```python
from build123d import *

# Parameters (mm, degrees)
SKETCH1_W                  = 50.8
SKETCH1_H                  = 76.2
BOSS_EXTRUDE1_DEPTH        = 1.5875
SKETCH2_W                  = 43.942
SKETCH2_H                  = 69.342
BOSS_EXTRUDE2_DEPTH        = 9.525
FILLET1_R                  = 6.35
CUT_EXTRUDE1_DEPTH         = 9.525
F_4_40_TAPPED_HOLE1_REACH  = 79.663
F_4_40_TAPPED_HOLE1_BORE_R = 1.1303
FILLET2_R                  = 1.5875


with BuildPart() as part:
    # Sketch1 → Boss-Extrude1 (new body)
    with BuildSketch(Plane.XY):
        Rectangle(SKETCH1_W, SKETCH1_H)
    extrude(amount=BOSS_EXTRUDE1_DEPTH)

    # Sketch2 → Boss-Extrude2 (add)
    with BuildSketch(Plane(origin=(0, 0, 0), x_dir=(-1, 0, 0), z_dir=(0, 0, -1))):
        Rectangle(SKETCH2_W, SKETCH2_H)
    extrude(amount=BOSS_EXTRUDE2_DEPTH)

    # Fillet1
    fillet1_edges = [part.edges().sort_by_distance(p)[0] for p in [
        (-21.971, -34.671, -4.7625),
        (-21.971, 34.671, -4.7625),
        (21.971, 34.671, -4.7625),
        (21.971, -34.671, -4.7625),
    ]]
    fillet(fillet1_edges, radius=FILLET1_R)

    # Sketch3 → Cut-Extrude1 (cut)
    with BuildSketch(Plane(origin=(0, 0, -9.525), x_dir=(-1, 0, 0), z_dir=(0, 0, -1))):
        with BuildLine():
            Line((-18.796, 28.321), (-18.796, -28.321))
            ThreePointArc((-18.796, -28.321), (-17.86606403, -30.56606403), (-15.621, -31.496))
            Line((-15.621, -31.496), (15.621, -31.496))
            ThreePointArc((15.621, -31.496), (17.86606403, -30.56606403), (18.796, -28.321))
            Line((18.796, -28.321), (18.796, 28.321))
            ThreePointArc((18.796, 28.321), (17.86606403, 30.56606403), (15.621, 31.496))
            Line((15.621, 31.496), (-15.621, 31.496))
            ThreePointArc((-15.621, 31.496), (-17.86606403, 30.56606403), (-18.796, 28.321))
        make_face()
    extrude(amount=-CUT_EXTRUDE1_DEPTH, mode=Mode.SUBTRACT)

    # 4-40 Tapped Hole1 bore → 4-40 Tapped Hole1 (cut, up to next)
    with BuildSketch(Plane(origin=(0, 34.671, 0), x_dir=(-1, 0, 0), z_dir=(0, 1, 0)), mode=Mode.PRIVATE) as f_4_40_tapped_hole1_sk1:
        with Locations((-9.525, -4.7625)):
            Circle(F_4_40_TAPPED_HOLE1_BORE_R)
    f_4_40_tapped_hole1_tool1 = extrude(f_4_40_tapped_hole1_sk1.sketch, amount=-F_4_40_TAPPED_HOLE1_REACH, mode=Mode.PRIVATE) & part.part
    # 4-40 Tapped Hole1 bore → 4-40 Tapped Hole1 (cut, up to next)
    with BuildSketch(Plane(origin=(0, 34.671, 0), x_dir=(-1, 0, 0), z_dir=(0, 1, 0)), mode=Mode.PRIVATE) as f_4_40_tapped_hole1_sk2:
        with Locations((9.525, -4.7625)):
            Circle(F_4_40_TAPPED_HOLE1_BORE_R)
    f_4_40_tapped_hole1_tool2 = extrude(f_4_40_tapped_hole1_sk2.sketch, amount=-F_4_40_TAPPED_HOLE1_REACH, mode=Mode.PRIVATE) & part.part
    f_4_40_tapped_hole1_1 = f_4_40_tapped_hole1_tool1.solids().sort_by_distance((9.525, 34.671, -4.7625))[0]
    add(f_4_40_tapped_hole1_1, mode=Mode.SUBTRACT)
    f_4_40_tapped_hole1_2 = f_4_40_tapped_hole1_tool2.solids().sort_by_distance((-9.525, 34.671, -4.7625))[0]
    add(f_4_40_tapped_hole1_2, mode=Mode.SUBTRACT)
    f_4_40_tapped_hole1 = f_4_40_tapped_hole1_1 + f_4_40_tapped_hole1_2  # 4-40 Tapped Hole1 as one shape, for the pattern or mirror that repeats it

    # Mirror1: 4-40 Tapped Hole1 across plane
    add(f_4_40_tapped_hole1.mirror(Plane.ZX), mode=Mode.SUBTRACT)

    # Fillet2
    fillet2_edges = [part.edges().sort_by_distance(p)[0] for p in [
        (25.4, -38.1, 0.79375),
        (-25.4, -38.1, 0.79375),
        (-25.4, 38.1, 0.79375),
        (25.4, 38.1, 0.79375),
    ]]
    fillet(fillet2_edges, radius=FILLET2_R)


solid = part.part
```
Design review of the part built by this model. Coordinates are the model's own, in mm. A direction names the side the tool comes from. Coordinates: 2 decimals unless noted, no trailing zeros. Order: outer loops, then holes, each group sorted by start corner. A loop starts at its lowest first (then second) coordinate and runs counter-clockwise, first axis right, second up. Notation, with made-up numbers: (74, 80) - (84, 80) arc R20 ccw to (84, 96) - close; hole circle Ø4 at (56, 78). An arc over 180 degrees is marked (long way). One line per question, with ' | ' between items.
Q1. Consider section C-C, the plane x = 17. Give the boundary of the cut face in (y, z) (1 decimal), then the cut area to 3 significant figures.
Answer key:
outline: (-38.1, 0) - (-34.5, 0) - (-34.5, -9.5) - (-31.2, -9.5) - (-31.2, 0) - (31.2, 0) - (31.2, -9.5) - (34.5, -9.5) - (34.5, 0) - (38.1, 0) - (38.1, 1.6) - (-38.1, 1.6) - close | area: 185 mm2
Q2. Consider section D-D, the plane y = 32.5. Give the boundary of the cut face in (x, z) (1 decimal).
Answer key:
outline: (-25.4, 0) - (-20.4, 0) - (-20.4, -9.5) - (20.4, -9.5) - (20.4, 0) - (25.4, 0) - (25.4, 1.6) - (-25.4, 1.6) - close; hole circle Ø2.3 at (-9.5, -4.8); hole circle Ø2.3 at (9.5, -4.8)
Q3. The part is to be moulded in two halves that separate along Z. For faces 1 (the cylindrical face through (10.654, 33.106, -4.713)), 2 (the cylindrical face through (-10.569, -33.106, -5.195)), 3 (the flat face through (0, 0, 0)), 4 (the cylindrical face through (-20.06, 32.86, -4.83)), say which applies: +Z half, -Z half, draft (parallel to the pull), parting line (faces both ways), or undercut.
Answer key:
face 1: undercut | face 2: undercut | face 3: -Z half | face 4: draft
Q4. Consider section B-B, the plane y = -19. Give the boundary of the cut face in (x, z) (1 decimal).
Answer key:
outline: (-25.4, 0) - (-22, 0) - (-22, -9.5) - (-18.8, -9.5) - (-18.8, 0) - (18.8, 0) - (18.8, -9.5) - (22, -9.5) - (22, 0) - (25.4, 0) - (25.4, 1.6) - (-25.4, 1.6) - close
Q5. To check wall thickness, follow line 1 along Y through (x, z) = (-5.5, -6.5); line 2 along X through (y, z) = (-22, -6); line 3 along Z through (x, y) = (-3.5, -25.5). State the ranges of each line that lie inside material, in increasing order.
Answer key:
line 1: y = -34.67 to -31.5, 31.5 to 34.67 | line 2: x = -21.97 to -18.8, 18.8 to 21.97 | line 3: z = 0 to 1.59
Q6. For faces 5 (the flat face through (0, 34.671, -5)), 6 (the cylindrical face through (-17.89, 30.54, -4.83)), 7 (the flat face through (0, -34.671, -5)), 8 (the cylindrical face through (-20.16, -32.76, -4.83)), 9 (the cylindrical face through (20.16, -32.76, -4.83)), list the 3-axis set-ups (+Z, -Z, +X, -X, +Y, -Y) from which the entire face can be reached by the end or side of a thin tool; tool diameter is ignored.
Answer key:
face 5: -Z, +X, -X, +Y | face 6: -Z | face 7: -Z, +X, -X, -Y | face 8: -Z, -X, -Y | face 9: -Z, +X, -Y
Q7. Consider section A-A, the plane z = -2. Give the boundary of the cut face in (x, y) (3 decimals), then the cut area to 3 significant figures.
Answer key:
outline: (-21.971, -28.321) arc R6.35 ccw to (-15.621, -34.671) - (15.621, -34.671) arc R6.35 ccw to (21.971, -28.321) - (21.971, 28.321) arc R6.35 ccw to (15.621, 34.671) - (-15.621, 34.671) arc R6.35 ccw to (-21.971, 28.321) - close; hole (-18.796, -28.321) arc R3.175 ccw to (-15.621, -31.496) - (15.621, -31.496) arc R3.175 ccw to (18.796, -28.321) - (18.796, 28.321) arc R3.175 ccw to (15.621, 31.496) - (-15.621, 31.496) arc R3.175 ccw to (-18.796, 28.321) - close | area: 653 mm2
Q8. Clearance check with flat-ended pins moving along their axes: pin 1 Ø1 at (y, z) = (22.5, -6.5) entering from +X; pin 2 Ø3 at (x, z) = (6.5, -5.5) entering from -Y; pin 3 Ø1 at (x, z) = (-4.5, -3.5) entering from +Y. State where each tip first meets the part, or that it passes through.
Answer key:
pin 1: stops at x = 21.97 | pin 2: stops at y = -34.67 | pin 3: stops at y = 34.67
